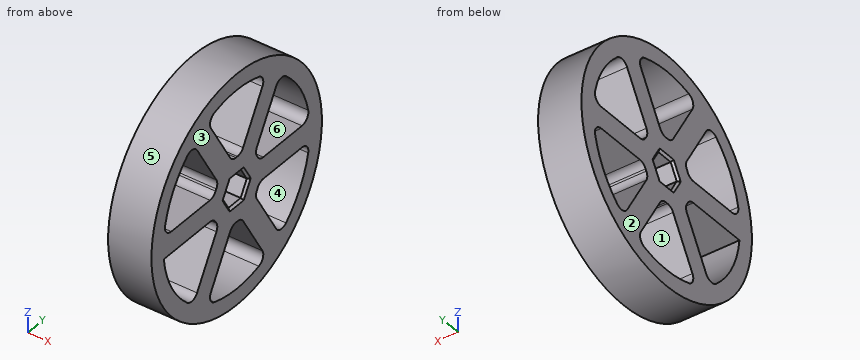
```python
from build123d import *

# Parameters (mm, degrees)
AXLE_PROFILE_R              = 9.525
WHEEL_HUB_DEPTH             = 12.7
WHEEL_RIM_REACH             = 16.892
SKETCH3_R                   = 33.9725
SKETCH3_R_2                 = 29.21
WHEEL_RIM_DIRECTION_2_REACH = 16.892
SKETCH4_W                   = 6.35
SKETCH4_H                   = 20.229743879
BOSS_EXTRUDE1_DEPTH         = 12.7
SPOKES_COUNT                = 6
SPOKE_FILLETS_R             = 2.54
SHAFT_CHAMFERS_SIZE         = 0.635


with BuildPart() as part:
    # Axle Profile → Wheel Hub (new body)
    with BuildSketch(Plane(origin=(0, 0, 0), x_dir=(0, 0, -1), z_dir=(1, 0, 0))):
        Circle(AXLE_PROFILE_R)
        Polygon((0, -4.8895), (4.234431212, -2.44475), (4.234431212, 2.44475), (0, 4.8895), (-4.234431212, 2.44475), (-4.234431212, -2.44475), align=None, mode=Mode.SUBTRACT)
    extrude(amount=WHEEL_HUB_DEPTH)

    # Wheel Rim: up to this face of the body (flat: up to its plane)
    wheel_rim_end = Plane(part.part.faces().sort_by_distance((0, 0, 9.255592316))[0])
    # Sketch3 → Wheel Rim (add, up to the picked face)
    with BuildSketch(Plane.ZY.offset(-6.35), mode=Mode.PRIVATE) as wheel_rim_sk1:
        with Locations(Location((0, 0, 0), (0, 0, 180))):
            Circle(SKETCH3_R)
        with Locations(Location((0, 0, 0), (0, 0, 180))):
            Circle(SKETCH3_R_2, mode=Mode.SUBTRACT)
    wheel_rim_tool1 = split(extrude(wheel_rim_sk1.sketch, amount=WHEEL_RIM_REACH, mode=Mode.PRIVATE), bisect_by=wheel_rim_end, keep=Keep.BOTH, mode=Mode.PRIVATE)
    add(wheel_rim_tool1.solids().sort_by(Axis((6.35, 0, 33.011613), (-1, 0, 0)))[0])

    # Wheel Rim direction 2: up to this face of the body (flat: up to its plane)
    wheel_rim_direction_2_end = Plane(part.part.faces().sort_by_distance((12.7, 0, 9.255592316))[0])
    # Sketch3 → Wheel Rim direction 2 (add, up to the picked face)
    with BuildSketch(Plane.ZY.offset(-6.35), mode=Mode.PRIVATE) as wheel_rim_direction_2_sk1:
        with Locations(Location((0, 0, 0), (0, 0, 180))):
            Circle(SKETCH3_R)
        with Locations(Location((0, 0, 0), (0, 0, 180))):
            Circle(SKETCH3_R_2, mode=Mode.SUBTRACT)
    wheel_rim_direction_2_tool1 = split(extrude(wheel_rim_direction_2_sk1.sketch, amount=-WHEEL_RIM_DIRECTION_2_REACH, mode=Mode.PRIVATE), bisect_by=wheel_rim_direction_2_end, keep=Keep.BOTH, mode=Mode.PRIVATE)
    add(wheel_rim_direction_2_tool1.solids().sort_by(Axis((6.35, 0, 33.011613), (1, 0, 0)))[0])

    # Sketch4 → Boss-Extrude1 (add)
    with BuildSketch(Plane(origin=(12.7, 0, 0), x_dir=(0, 0, -1), z_dir=(1, 0, 0))):
        with Locations((0, 19.095128061)):
            Rectangle(SKETCH4_W, SKETCH4_H)
    boss_extrude1 = extrude(amount=-BOSS_EXTRUDE1_DEPTH)

    # Spokes: Boss-Extrude1 ×6 about axis
    spokes_axis = Axis((0, 0, 0), (1, 0, 0))
    for i in range(1, SPOKES_COUNT):
        add(boss_extrude1.rotate(spokes_axis, i * 360 / SPOKES_COUNT))

    # Spoke Fillets
    spoke_fillets_edges = [part.edges().sort_by_distance(p)[0] for p in [
        (6.35, 7.239758718, -6.189629933),
        (6.35, 1.740497404, -9.364629933),
        (6.35, -1.740497404, -9.364629933),
        (6.35, -7.239758718, -6.189629933),
        (6.35, -8.980256121, -3.175),
        (6.35, -8.980256121, 3.175),
        (6.35, -7.239758718, 6.189629933),
        (6.35, -1.740497404, 9.364629933),
        (6.35, 1.740497404, 9.364629933),
        (6.35, 7.239758718, 6.189629933),
        (6.35, 8.980256121, 3.175),
        (6.35, 8.980256121, -3.175),
        (9.525, 29.036932948, -3.175),
        (9.525, 29.036932948, 3.175),
        (3.175, 17.268097131, 23.559221581),
        (3.175, 11.768835817, 26.734221581),
        (9.525, -11.768835817, 26.734221581),
        (9.525, -17.268097131, 23.559221581),
        (9.525, -29.036932948, 3.175),
        (3.175, -17.268097131, -23.559221581),
        (3.175, -11.768835817, -26.734221581),
        (9.525, 11.768835817, -26.734221581),
        (3.175, 17.268097131, -23.559221581),
    ]]
    fillet(spoke_fillets_edges, radius=SPOKE_FILLETS_R)

    # Shaft Chamfers
    shaft_chamfers_edges = [part.edges().sort_by_distance(p)[0] for p in [
        (0, 0, -4.234431212),
        (0, 3.667125, -2.117215606),
        (0, 3.667125, 2.117215606),
        (0, 0, 4.234431212),
        (12.7, -3.667125, 2.117215606),
        (12.7, -3.667125, -2.117215606),
        (12.7, 0, -4.234431212),
        (12.7, 3.667125, -2.117215606),
        (12.7, 3.667125, 2.117215606),
        (12.7, 0, 4.234431212),
        (0, -3.667125, 2.117215606),
        (0, -3.667125, -2.117215606),
    ]]
    chamfer(shaft_chamfers_edges, length=SHAFT_CHAMFERS_SIZE)


solid = part.part
```
Check sheet for the modelled part. Datum: model origin and axes. Units: mm. Face numbers are marked on the shaded views. A direction names the side the tool comes from. Round coordinates to 2 decimals unless told otherwise and drop trailing zeros. Loops run counter-clockwise (first coordinate to the right, second up) from the corner with the lowest first, then second, coordinate; pieces in that order, holes last. Notation, with made-up numbers: (-12.5, 1) -> (36.5, 1) arc R23 ccw to (36.5, 33) -> close; hole circle Ø5 at (-32, 56). An arc over 180 degrees is marked (long way). Write item = value, one per line. Start each with the question number.
1) Sectioned sample at B-B, the plane z = -27. Record the cut outline in (x, y).
2) Set-up check for the marked faces 1 and 2: record each of +Z, -Z, +X, -X, +Y, -Y from which the full face is reachable in a straight line by a thin tool's end or side.
3) Sectioned sample at A-A, the plane y = 22. Record the cut outline in (x, z) (3 decimals).
4) Gauge pin test, flat ends, axial feed: pin 1 Ø1.5 at (x, z) = (11, -19) entering from +Y; pin 2 Ø4 at (x, y) = (3.5, 22) entering from +Z; pin 3 Ø3 at (x, y) = (2.5, -23.5) entering from +Z. Record the tip position at first contact, or that the pin passes through.
5) Release check for a two-part mould opening along Y. For the marked faces 3, 4, 5 and 6 record: released by +Y, released by -Y, zero draft, split by the parting line, or undercut.
6) Thickness scan on probe 1 along Y at (x, z) = (11.5, -7.5); probe 2 along Z at (x, y) = (2.5, -18) (3 decimals); probe 3 along Z at (x, y) = (5.25, -17) (3 decimals). Record the ranges inside material, lowest first.
7) Sectioned sample at D-D, the plane z = -1. Record the cut outline in (x, y) (3 decimals).
8) Sectioned sample at C-C, the plane x = 9.5. State how many separate pieces and enclosed holes the cut face has, plus the area to 3 significant figures.
Results are:
q1.outline = (0, -20.62) -> (12.7, -20.62) -> (12.7, -10.06) -> (0, -10.06) -> close; (0, 10.06) -> (12.7, 10.06) -> (12.7, 20.62) -> (0, 20.62) -> close
q2.face_1 = +X, -X
q2.face_2 = +Z, -Z, -X, +Y, -Y
q3.outline = (0, -25.887) -> (12.7, -25.887) -> (12.7, -19.215) -> (0, -19.215) -> close; (0, -3.175) -> (12.7, -3.175) -> (12.7, 3.175) -> (0, 3.175) -> close; (0, 19.215) -> (12.7, 19.215) -> (12.7, 25.887) -> (0, 25.887) -> close
q4.pin_1 = 28.65
q4.pin_2 = 27.46
q4.pin_3 = 25.89
q5.face_3 = zero draft
q5.face_4 = undercut
q5.face_5 = split by the parting line
q5.face_6 = undercut
q6.probe_1 = -33.13 to -28.23, -8 to 8, 28.23 to 33.13
q6.probe_2 = -28.812 to -22.243, -3.175 to 3.175, 22.243 to 28.812
q6.probe_3 = -29.413 to -22.048, -3.175 to 3.175, 22.048 to 29.413
q7.outline = (0, -33.958) -> (12.7, -33.958) -> (12.7, -5.045) -> (12.065, -4.312) -> (0.635, -4.312) -> (0, -5.045) -> close; (0, 5.045) -> (0.635, 4.312) -> (12.065, 4.312) -> (12.7, 5.045) -> (12.7, 33.958) -> (0, 33.958) -> close
q8.separate_pieces = 1
q8.enclosed_holes = 7
q8.area = 1,950 mm^2
